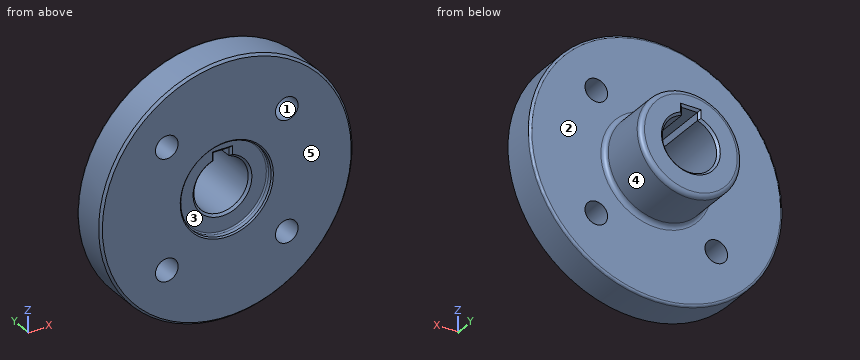
from build123d import *

# Parameters (mm, degrees)
F2_W     = 7
F2_H     = 7
F3_DEPTH = 40.001
F5_D     = 10
F6_SIZE  = 1
F7_SIZE  = 0.6
F8_R     = 0.6
F9_SIZE  = 1
F10_R    = 1
F11_R    = 2


with BuildPart() as f1:
    # F0 (on Right) → F1 (revolve)
    with BuildSketch(Plane.YZ):
        Polygon((0, 56), (0, 20), (3, 20), (3, 12), (40, 12), (40, 22.5), (16, 22.5), (16, 56), align=None)
    revolve(axis=Axis((0, 11.147524, 0), (0, 1, 0)))

    # F2 (on face) → F3 (cut, through all)
    with BuildSketch(Plane(origin=(0, 40, 0), x_dir=(-1, 0, 0), z_dir=(0, 1, 0))):
        with Locations((0, 11.5)):
            Rectangle(F2_W, F2_H)
    extrude(amount=-F3_DEPTH, mode=Mode.SUBTRACT)

    # F5 (through all)
    with Locations(Plane(origin=(0, 16, 0), x_dir=(-1, 0, 0), z_dir=(0, 1, 0))):
        with Locations((26.516504, 26.516504), (-26.516504, 26.516504), (-26.516504, -26.516504), (26.516504, -26.516504)):
            Hole(F5_D / 2)

    # F6
    f6_edges = [f1.edges().sort_by_distance(p)[0] for p in [
        (0, 3, -12),
        (-3.5, 40, 13.23912),
        (0, 40, 15),
        (3.5, 40, 13.23912),
        (-3.5, 3, 13.23912),
        (0, 40, -12),
        (3.5, 3, 13.23912),
        (0, 3, 15),
    ]]
    chamfer(f6_edges, length=F6_SIZE)

    # F7
    f7_edges = [f1.edges().sort_by_distance(p)[0] for p in [
        (0, 0, -20),
    ]]
    chamfer(f7_edges, length=F7_SIZE)

    # F8
    f8_edges = [f1.edges().sort_by_distance(p)[0] for p in [
        (0, 3, -20),
    ]]
    fillet(f8_edges, radius=F8_R)

    # F9
    f9_edges = [f1.edges().sort_by_distance(p)[0] for p in [
        (0, 0, -56),
    ]]
    chamfer(f9_edges, length=F9_SIZE)

    # F10
    f10_edges = [f1.edges().sort_by_distance(p)[0] for p in [
        (0, 16, -56),
    ]]
    fillet(f10_edges, radius=F10_R)

    # F11
    f11_edges = [f1.edges().sort_by_distance(p)[0] for p in [
        (0, 40, -22.5),
        (0, 16, -22.5),
    ]]
    fillet(f11_edges, radius=F11_R)


solid = f1.part
Geometry: final body of the model. Coordinates: model frame, mm. Face numbers are marked on the shaded views. A direction names the side the tool comes from. Coordinates: 2 decimals unless noted, no trailing zeros. Loops run counter-clockwise (first coordinate to the right, second up) from the corner with the lowest first, then second, coordinate; pieces in that order, holes last. Notation, with made-up numbers: M -27,66.5 L 7,66.5 A18 ccw 7,74.5 Z; hole C 66,-10.75 d10. An arc over 180 degrees is marked long. One line per item, written item: value. Start each with the question number.
1) Reachability of the marked faces 1 and 2 from +Z, -Z, +X, -X, +Y, -Y: full face, straight path, thin tool, end or side. Return the list, or none.
2) Material intervals for L1, parallel to X at y = 23, z = 0; L2, parallel to X at y = 8, z = -27.5; L3, parallel to Z at x = -0.5, y = 21, sorted ascending. Write a range as from..to.
3) Cut plane C-C (y = 25.5). Return loops of the section in (x, z), then the cut area to 3 significant figures.
4) Pin query (flat end, axial travel): P1, Ø2, axis at x = -5.5, y = 30, coming from the -Z side; P2, Ø4, axis at y = 23, z = 13, coming from the -X side; P3, Ø4, axis at x = 10, y = 34.5, coming from the -Z side. Return the tip coordinate at first contact, or that it passes through.
5) Draft query along Z for the marked faces 3, 4 and 5. Return one class per face: released by +Z, released by -Z, zero draft, split by the parting line, or undercut.
6) Cut plane D-D (y = 12). Return loops of the section in (x, z), then the cut area to 3 significant figures.
Evaluation:
1. face 1: +Y, -Y
1. face 2: +Y
2. L1: -22.5..-12, 12..22.5
2. L2: -48.78..-31.42, -21.61..21.61, 31.42..48.78
2. L3: -22.49..-11.99, 15..22.49
3. outline: C 0,0 d45; hole M -3.5,11.48 A12 ccw long 3.5,11.48 L 3.5,15 L -3.5,15 Z
3. area: 1,120 mm^2
4. P1: z = -22.05
4. P2: x = -19.63
4. P3: z = -21.03
5. face 3: undercut
5. face 4: split by the parting line
5. face 5: zero draft
6. outline: C 0,0 d112; hole C -26.52,-26.52 d10; hole C -26.52,26.52 d10; hole M -3.5,11.48 A12 ccw long 3.5,11.48 L 3.5,15 L -3.5,15 Z; hole C 26.52,-26.52 d10; hole C 26.52,26.52 d10
6. area: 9,060 mm^2
